Source: CAD feature listing. Evaluate the final solid. Frame: model axes, mm. A direction names the side the tool comes from. Round coordinates to 2 decimals unless told otherwise and drop trailing zeros. Loops run counter-clockwise (first coordinate to the right, second up) from the corner with the lowest first, then second, coordinate; pieces in that order, holes last. Notation, with made-up numbers: M 40,73 L 61,73 A20 ccw 61,77 Z; hole C -29.5,61 d7. An arc over 180 degrees is marked long. Answer as CSV lines item,"result". Start each with the question number.
```python
from build123d import *

# Parameters (mm, degrees)
F0_R     = 19.8
F1_DEPTH = 16
F3_DEPTH = 3
F4_R     = 19.8
F4_R_2   = 6
F5_DEPTH = 8
F7_D     = 9
F8_R     = 6
F8_R_2   = 4.5
F9_DEPTH = 2


with BuildPart() as f1:
    # F0 (on Top) → F1 (new body)
    with BuildSketch(Plane.XY):
        Circle(F0_R)
    extrude(amount=F1_DEPTH)

    # F2 (on face) → F3 (cut)
    with BuildSketch(Plane.XY.offset(16)):
        with BuildLine():
            Line((-10.95, -16.4965905568), (-10.95, 16.4965905568))
            ThreePointArc((-10.95, 16.4965905568), (-19.8, 0), (-10.95, -16.4965905568))
        make_face()
        with BuildLine():
            ThreePointArc((19.8, 0), (17.4477792283, 9.3602884571), (10.95, 16.4965905568))
            Line((10.95, 16.4965905568), (10.95, -16.4965905568))
            ThreePointArc((10.95, -16.4965905568), (17.4477792283, -9.3602884571), (19.8, 0))
        make_face()
    extrude(amount=-F3_DEPTH, mode=Mode.SUBTRACT)

    # F4 (on face) → F5 (cut)
    with BuildSketch(Plane(origin=(0, 0, 0), x_dir=(1, 0, 0), z_dir=(0, 0, -1))):
        Circle(F4_R)
        Circle(F4_R_2, mode=Mode.SUBTRACT)
    extrude(amount=-F5_DEPTH, mode=Mode.SUBTRACT)

    # F7 (through all)
    with Locations(Plane(origin=(0, 0, 0), x_dir=(1, 0, 0), z_dir=(0, 0, -1))):
        with Locations((0, 0)):
            Hole(F7_D / 2)

    # F8 (on face) → F9 (cut)
    with BuildSketch(Plane.XY.offset(16)):
        Circle(F8_R)
        Circle(F8_R_2, mode=Mode.SUBTRACT)
    extrude(amount=-F9_DEPTH, mode=Mode.SUBTRACT)


solid = f1.part
```
1) Section A-A, the plane x = 0. Return loops of the section in (y, z), and give its area (3 significant figures).
2) Contact query for flat-ended pins moving along their axis: pin 1 Ø4.5 at (x, y) = (-16.5, 3.5) entering from +Z; pin 2 Ø8 at (y, z) = (-6.5, 8.5) entering from -X; pin 3 Ø4 at (x, z) = (7.5, 8.5) entering from -Y. Output: stop coordinate, or through.
3) Ray query, line 1 along Y through (x, z) = (0, 9.75); line 2 along Y through (x, z) = (0, 14.85); line 3 along Z through (x, y) = (-9, 5). Return the intervals inside material, ascending.
4) Section C-C, the plane z = 5.75. Return loops of the section in (x, y), and give its area (3 significant figures).
5) Mould query, pull axis X, two halves, no side actions, for faces 1 (the flat face through (5, -4, 16)), 2 (the flat face through (-1.4, 4.5, 14)), 3 (the flat face through (10.95, 0, 15)). Classes: pulls with the +X half, pulls with the -X half, needs draft (parallel to the pull), parting line crosses it, or undercut.
6) Section B-B, the plane y = 0. Return loops of the section in (x, z).
7) Access query for faces 4 (the flat face through (-5, 4, 8)), 5 (the flat face through (14, 0, 13)), 6 (the flat face through (-14, 0, 13)). Directions: +Z, -Z, +X, -X, +Y, -Y. A direction counts if a zero-diameter tool reaches every point of the face in a straight line with its end or side. Return the directions, or none.
8) Section D-D, the plane y = -6.5. Return loops of the section in (x, z).
Findings below:
1,outline,"M -19.8,8 L -6,8 L -6,0 L -4.5,0 L -4.5,14 L -6,14 L -6,16 L -19.8,16 Z; M 4.5,0 L 6,0 L 6,8 L 19.8,8 L 19.8,16 L 6,16 L 6,14 L 4.5,14 Z"
1,area,"263 mm²"
2,pin 1,"z = 13"
2,pin 2,"x = -19.64"
2,pin 3,"y = -19.02"
3,line 1,"-19.8 to -4.5, 4.5 to 19.8"
3,line 2,"-19.8 to -6, 6 to 19.8"
3,line 3,"8 to 16"
4,outline,"C 0,0 d12; hole C 0,0 d9"
4,area,"49.5 mm²"
5,face 1,"needs draft"
5,face 2,"undercut"
5,face 3,"pulls with the +X half"
6,outline,"M -19.8,8 L -6,8 L -6,0 L -4.5,0 L -4.5,14 L -6,14 L -6,16 L -10.95,16 L -10.95,13 L -19.8,13 Z; M 4.5,0 L 6,0 L 6,8 L 19.8,8 L 19.8,13 L 10.95,13 L 10.95,16 L 6,16 L 6,14 L 4.5,14 Z"
7,face 4,"-Z"
7,face 5,"+Z, +X, +Y, -Y"
7,face 6,"+Z, -X, +Y, -Y"
8,outline,"M -18.7,8 L 18.7,8 L 18.7,13 L 10.95,13 L 10.95,16 L -10.95,16 L -10.95,13 L -18.7,13 Z"
